For this review, take the finished solid that the model builds, in its own axes (mm). A direction names the side the tool comes from. Give positions to 0.01 mm unless a question says otherwise; leave off trailing zeros. Loops run counter-clockwise (first coordinate to the right, second up) from the corner with the lowest first, then second, coordinate; pieces in that order, holes last. Notation, with made-up numbers: (5, 66) - (30, 66) arc R32 ccw to (30, 103) - close; hole circle Ø4 at (-14, 88). An arc over 180 degrees is marked (long way). Put each result on its own line as item: value. Start each with the question number.
from build123d import *

# Parameters (mm, degrees)
SKETCH_R        = 18
PAD_DEPTH       = 10
SKETCH001_R     = 16.1
POCKET_DEPTH    = 1.6
POCKET001_DEPTH = 5
SKETCH004_R     = 3.5
POCKET002_DEPTH = 3.5


with BuildPart() as part:
    # Sketch → Pad (new body)
    with BuildSketch(Plane.XY):
        Circle(SKETCH_R)
    extrude(amount=PAD_DEPTH)

    # Sketch001 → Pocket (cut)
    with BuildSketch(Plane.XY.offset(10)):
        with Locations((0.069364, -0.076041)):
            Circle(SKETCH001_R)
    extrude(amount=-POCKET_DEPTH, mode=Mode.SUBTRACT)

    # Sketch003 → Pocket001 (cut)
    with BuildSketch(Plane.XY.offset(10)):
        with BuildLine():
            ThreePointArc((0, 6), (-6, 0), (0, -6))
            Line((0, -6), (30, -6))
            ThreePointArc((30, -6), (36, 0), (30, 6))
            Line((0, 6), (30, 6))
        make_face()
    extrude(amount=-POCKET001_DEPTH, mode=Mode.SUBTRACT)

    # Sketch004 → Pocket002 (cut)
    with BuildSketch(Plane(origin=(0, 0, 0), x_dir=(1, 0, 0), z_dir=(0, 0, -1))):
        Circle(SKETCH004_R)
    extrude(amount=-POCKET002_DEPTH, mode=Mode.SUBTRACT)


solid = part.part
1) Insertion check: P1, Ø6, axis at x = -5, z = 4, coming from the +Y side; P2, Ø5, axis at x = -5, z = 8, coming from the -Y side; P3, Ø2, axis at x = 1, y = 0, coming from the -Z side. Each pin has a flat end and moves straight along its axis. Give the tip position at first contact, or say it passes through.
2) Take a section at A-A on y = -9.5. State the section outline as (x, z) points.
3) Wall thickness on probe 1 along Z at (x, y) = (-6.5, 0.5); probe 2 along X at (y, z) = (8.5, 9.5); probe 3 along X at (y, z) = (14, 9.5): over which ranges is each line inside the solid? List them lowest first.
4) Take a section at B-B on x = -6.5. State the section outline as (y, z) points, and give its area (3 significant figures).
5) Machinability: for faces 1 (the flat face through (6, 0, 5)), 2 (the flat face through (0, -4, 0)), 3 (the flat face through (0, 0, 3.5)), 4 (the cylindrical face through (-16.02, 0.46, 9.21)), which of the approach directions +Z, -Z, +X, -X, +Y, -Y give a long, thin tool a straight path to every point of the face, cutting with its end or side? Answer none if there is none.
6) Take a section at D-D on z = 6.75. State the section outline as (x, y) points, and give its area (3 significant figures).
7) Take a section at C-C on z = 2.5. State the section outline as (x, y) points.
8) Mouldability with a two-part tool opening along Y and no side actions: class faces 5 (the flat face through (-16.14, 1.42, 10)), 6 (the flat face through (-8, 0, 8.4)), 7 (the flat face through (8, 6, 7)), 8 (the cylindrical face through (-17.983, 0.791, 4.93)) as released by +Y, released by -Y, zero draft, split by the parting line, or undercut.
Answers follow:
1. P1: y = 17.89
1. P2: y = -17.83
1. P3: z = 3.5
2. outline: (-15.29, 0) - (15.29, 0) - (15.29, 10) - (13.12, 10) - (13.12, 8.4) - (-12.98, 8.4) - (-12.98, 10) - (-15.29, 10) - close
3. probe 1: 0 to 8.4
3. probe 2: -15.87 to -13.56, 13.7 to 15.87
3. probe 3: -11.31 to -7.75, 7.88 to 11.31
4. outline: (-16.79, 0) - (16.79, 0) - (16.79, 10) - (14.62, 10) - (14.62, 8.4) - (-14.77, 8.4) - (-14.77, 10) - (-16.79, 10) - close
4. area: 289 mm2
5. face 1: +Z, +X
5. face 2: -Z, +X, -X, +Y, -Y
5. face 3: -Z
5. face 4: +Z
6. outline: (0, -6) arc R6 cw to (0, 6) - (16.97, 6) arc R18 ccw (long way) to (16.97, -6) - close
6. area: 749 mm2
7. outline: circle Ø36 at (0, 0); hole circle Ø7 at (0, 0)
8. face 5: zero draft
8. face 6: undercut
8. face 7: undercut
8. face 8: split by the parting line
